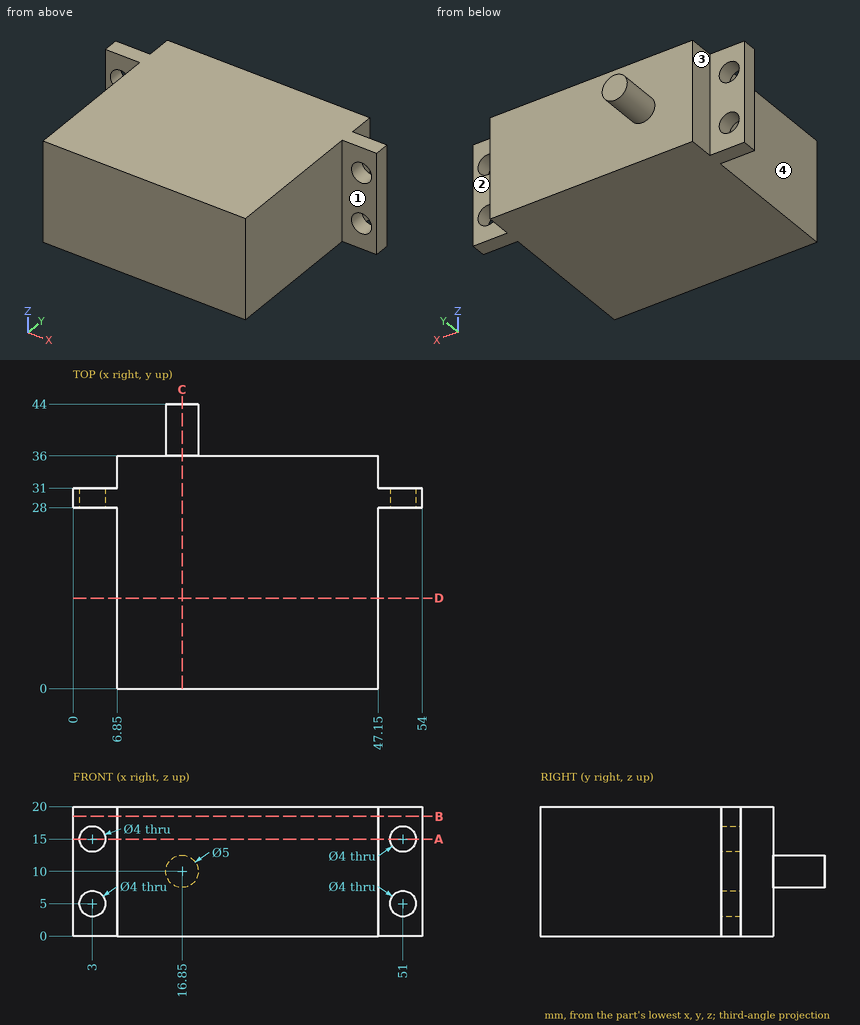
Check sheet for the drawn part. Datum: minimum x, y, z corner. Units: mm. A direction names the side the tool comes from. Round coordinates to 2 decimals unless told otherwise and drop trailing zeros. Order: outer loops, then holes, each group sorted by start corner. A loop starts at its lowest first (then second) coordinate and runs counter-clockwise, first axis right, second up.
1) Scan lines: line 1 (X direction, y = 30.15, z = 5); line 2 (X direction, y = 26.5, z = 2.5); line 3 (Y direction, x = 52, z = 3). Record each from-to range of solid material in increasing order.
2) Section check C-C (x = 16.85). Record the boundary of the cut face in (y, z).
3) Tool access check on the marked faces 1, 2, 3 and 4. Record the directions out of +Z, -Z, +X, -X, +Y, -Y that give a thin tool (end or side, any length) a straight path to the whole face; none if there is none.
4) Section check B-B (z = 18.5). Record the boundary of the cut face in (x, y), and give its area (3 significant figures).
5) Section check D-D (y = 14). Record the boundary of the cut face in (x, z), and give its area (3 significant figures).
6) Section check A-A (z = 15). Record the boundary of the cut face in (x, y), and give its area (3 significant figures).
7) Go/stop test with flat-tipped pins: pin 1 Ø2 at (x, y) = (16, 17) entering from -Z; pin 2 Ø5.5 at (y, z) = (34, 13.5) entering from -X; pin 3 Ø3 at (y, z) = (36.5, 16) entering from +X; pin 4 Ø3.5 at (x, z) = (49.5, 7) entering from -Y. Record where each tip stops, or that it passes through.
Result:
1. line 1: x = 0 to 1, 5 to 49, 53 to 54
1. line 2: x = 6.85 to 47.15
1. line 3: y = 28 to 31
2. outline: (0, 0) - (36, 0) - (36, 7.5) - (44, 7.5) - (44, 12.5) - (36, 12.5) - (36, 20) - (0, 20) - close
3. face 1: +Z, -Z, +X, -Y
3. face 2: +Z, -Z, +X, +Y
3. face 3: +Z, -Z, -X, +Y
3. face 4: +Z, -Z, -X, -Y
4. outline: (0, 28) - (6.85, 28) - (6.85, 0) - (47.15, 0) - (47.15, 28) - (54, 28) - (54, 31) - (47.15, 31) - (47.15, 36) - (6.85, 36) - (6.85, 31) - (0, 31) - close
4. area: 1,490 mm2
5. outline: (6.85, 0) - (47.15, 0) - (47.15, 20) - (6.85, 20) - close
5. area: 806 mm2
6. outline: (0, 28) - (1, 28) - (1, 31) - (0, 31) - close; (5, 28) - (6.85, 28) - (6.85, 0) - (47.15, 0) - (47.15, 28) - (49, 28) - (49, 31) - (47.15, 31) - (47.15, 36) - (6.85, 36) - (6.85, 31) - (5, 31) - close; (53, 28) - (54, 28) - (54, 31) - (53, 31) - close
6. area: 1,470 mm2
7. pin 1: stops at z = 0
7. pin 2: stops at x = 6.85
7. pin 3: stops at x = 47.15
7. pin 4: stops at y = 28
